Work out the finished part from the listing and answer in its coordinate system (mm). Face numbers are marked on the shaded views. A direction names the side the tool comes from. Round coordinates to 2 decimals unless told otherwise and drop trailing zeros. Loops run counter-clockwise (first coordinate to the right, second up) from the corner with the lowest first, then second, coordinate; pieces in that order, holes last.
from build123d import *

# Parameters (mm, degrees)
SKETCH1_R           = 8
BOSS_EXTRUDE1_DEPTH = 10
SKETCH2_W           = 3.7
SKETCH2_H           = 20
BOSS_EXTRUDE2_DEPTH = 18.7
SKETCH3_R           = 1.55
CUT_EXTRUDE1_DEPTH  = 18.7
BOSS_EXTRUDE3_START = -5
SKETCH4_R           = 8
SKETCH4_R_2         = 6
BOSS_EXTRUDE3_DEPTH = 5
CHAMFER1_SIZE       = 1
FILLET1_R           = 0.5


with BuildPart() as part:
    # Sketch1 → Boss-Extrude1 (new body)
    with BuildSketch(Plane.XY):
        with BuildLine():
            Line((-9.35, -4.920052783), (-9.35, -17.5))
            Line((-9.35, -17.5), (9.35, -17.5))
            Line((9.35, -17.5), (9.35, -4.920052783))
            ThreePointArc((9.35, -4.920052783), (0, 19.5), (-9.35, -4.920052783))
        make_face()
        with Locations((0, 5.5)):
            Circle(SKETCH1_R, mode=Mode.SUBTRACT)
    extrude(amount=BOSS_EXTRUDE1_DEPTH)

    # Sketch2 → Boss-Extrude2 (add)
    with BuildSketch(Plane(origin=(9.35, 0, 0), x_dir=(0, 0, -1), z_dir=(1, 0, 0))):
        with Locations((-5, -17.5)):
            Rectangle(SKETCH2_W, SKETCH2_H)
    extrude(amount=-BOSS_EXTRUDE2_DEPTH)

    # Sketch3 → Cut-Extrude1 (cut)
    with BuildSketch(Plane.XY.offset(6.85)):
        with Locations((0, -22.5)):
            Circle(SKETCH3_R)
    extrude(amount=-CUT_EXTRUDE1_DEPTH, mode=Mode.SUBTRACT)

    # Sketch4 → Boss-Extrude3 (add)
    with BuildSketch(Plane.XY.offset(10).offset(BOSS_EXTRUDE3_START)):
        with Locations((0, 5.5)):
            Circle(SKETCH4_R)
        with Locations((0, 5.5)):
            Circle(SKETCH4_R_2, mode=Mode.SUBTRACT)
    extrude(amount=BOSS_EXTRUDE3_DEPTH)

    # Chamfer1
    chamfer1_edges = [part.edges().sort_by_distance(p)[0] for p in [
        (-6, 5.5, 5),
    ]]
    chamfer(chamfer1_edges, length=CHAMFER1_SIZE)

    # Fillet1
    fillet1_edges = [part.edges().sort_by_distance(p)[0] for p in [
        (-8, 5.5, 0),
    ]]
    fillet(fillet1_edges, radius=FILLET1_R)


solid = part.part
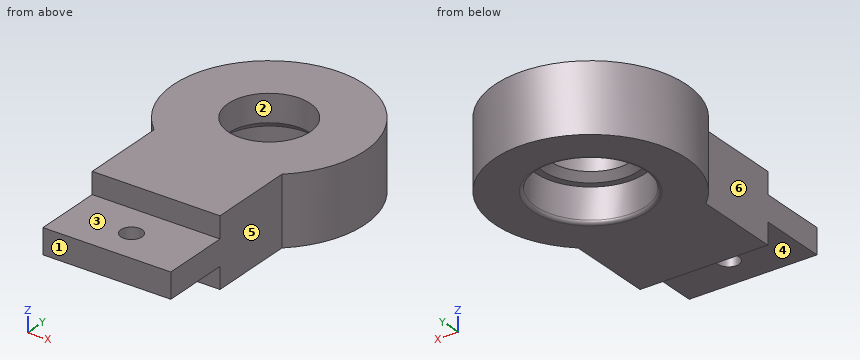
Item 1: Determine the mould class of the marked faces 1, 2 and 3 for opening direction Y: pulls with the +Y half, pulls with the -Y half, needs draft (parallel to the pull), parting line crosses it, or undercut.
Item 2: For the marked faces 4, 5 and 6, determine the directions among +Z, -Z, +X, -X, +Y, -Y from which every point of the face is accessible in a straight line to the end or side of a thin tool.
Item 3: Section C-C, the plane z = 4.5 is taken. Give the vertices of the cut face in (x, y), plus the area to 3 significant figures.
Item 4: Section B-B, the plane x = 0 is taken. Give the vertices of the cut face in (y, z).
Item 5: Section D-D, the plane z = 1.5 is taken. Give the vertices of the cut face in (x, y), plus the area to 3 significant figures.
Item 6: Straight lines are drawn through the part: line 1 (Y direction, x = 0, z = 3.7); line 2 (Y direction, x = 0, z = 7.55); line 3 (Y direction, x = 0, z = 2). For each, find the intervals that lie inside material, in ascending order.
Item 7: Section A-A, the plane y = -22.5 is taken. Give the vertices of the cut face in (x, z), plus the area to 3 significant figures.
Item 8: Each of these flat-tipped pins is pushed along its axis until it touches: P1, Ø5, axis at x = -3.5, y = -24, coming from the -Z side; P2, Ø3, axis at y = -19.5, z = 5, coming from the -X side; P3, Ø5, axis at x = 0, y = -22.5, coming from the +Z side; P4, Ø9.5, axis at x = 0, y = 5.5, coming from the -Z side. Where does it stop, or does it pass through?
Answer below:
1. face 1: pulls with the -Y half
1. face 2: undercut
1. face 3: needs draft
2. face 4: -Z, +X, -X, -Y
2. face 5: +Z, -Z, +X, -Y
2. face 6: +Z, -Z, -X, -Y
3. outline: (-9.35, -27.5) - (9.35, -27.5) - (9.35, -4.92) arc R14 ccw (long way) to (-9.35, -4.92) - close; hole circle Ø16 at (0, 5.5); hole circle Ø3.1 at (0, -22.5)
3. area: 783 mm2
4. outline: (-27.5, 3.15) - (-24.05, 3.15) - (-24.05, 6.85) - (-27.5, 6.85) - close; (-20.95, 3.15) - (-17.5, 3.15) - (-17.5, 0) - (-3, 0) arc R0.5 ccw to (-2.5, 0.5) - (-2.5, 5) - (-1.5, 5) - (-0.5, 6) - (-0.5, 10) - (-17.5, 10) - (-17.5, 6.85) - (-20.95, 6.85) - close; (11.5, 6) - (12.5, 5) - (13.5, 5) - (13.5, 0.5) arc R0.5 ccw to (14, 0) - (19.5, 0) - (19.5, 10) - (11.5, 10) - close
5. outline: (-9.35, -17.5) - (9.35, -17.5) - (9.35, -4.92) arc R14 ccw (long way) to (-9.35, -4.92) - close; hole circle Ø16 at (0, 5.5)
5. area: 604 mm2
6. line 1: y = -27.5 to -24.05, -20.95 to -2.5, 13.5 to 19.5
6. line 2: y = -17.5 to -0.5, 11.5 to 19.5
6. line 3: y = -17.5 to -2.5, 13.5 to 19.5
7. outline: (-9.35, 3.15) - (-1.55, 3.15) - (-1.55, 6.85) - (-9.35, 6.85) - close; (1.55, 3.15) - (9.35, 3.15) - (9.35, 6.85) - (1.55, 6.85) - close
7. area: 57.7 mm2
8. P1: stops at z = 3.15
8. P2: stops at x = -9.35
8. P3: stops at z = 6.85
8. P4: passes through
